```python
from build123d import *

# Parameters (mm, degrees)
SKETCH1_W           = 43.5
SKETCH1_H           = 42.15
SKETCH1_R           = 4
SKETCH1_R_2         = 1
BOSS_EXTRUDE1_DEPTH = 1
BOSS_EXTRUDE2_DEPTH = 3.8
BOSS_EXTRUDE5_DEPTH = 12.8
FILLET1_R           = 1
SKETCH3_R           = 1
CUT_EXTRUDE1_DEPTH  = 63.12336517


with BuildPart() as part:
    # Sketch1 → Boss-Extrude1 (new body)
    with BuildSketch(Plane(origin=(0, 0, 0), x_dir=(1, 0, 0), z_dir=(0, 1, 0))):
        with Locations((21.75, 21.075)):
            Rectangle(SKETCH1_W, SKETCH1_H)
        with Locations(Location((21.75, 21.075, 0), (0, 0, 270))):
            Circle(SKETCH1_R, mode=Mode.SUBTRACT)
        with Locations(Location((21.75, 30.775, 0), (0, 0, 270))):
            Circle(SKETCH1_R, mode=Mode.SUBTRACT)
        with Locations(Location((21.75, 11.375, 0), (0, 0, 90))):
            Circle(SKETCH1_R, mode=Mode.SUBTRACT)
        with Locations(Location((8.55, 21.075, 0), (0, 0, 270))):
            Circle(SKETCH1_R_2, mode=Mode.SUBTRACT)
        with Locations(Location((8.55, 30.725, 0), (0, 0, 270))):
            Circle(SKETCH1_R_2, mode=Mode.SUBTRACT)
        with Locations(Location((8.55, 11.425, 0), (0, 0, 90))):
            Circle(SKETCH1_R_2, mode=Mode.SUBTRACT)
        with Locations(Location((34.95, 11.425, 0), (0, 0, 270))):
            Circle(SKETCH1_R_2, mode=Mode.SUBTRACT)
        with Locations(Location((34.95, 21.075, 0), (0, 0, 90))):
            Circle(SKETCH1_R_2, mode=Mode.SUBTRACT)
        with Locations(Location((34.95, 30.725, 0), (0, 0, 90))):
            Circle(SKETCH1_R_2, mode=Mode.SUBTRACT)
        with Locations(Location((17.012384566, 35.512615434, 0), (0, 0, 270))):
            Circle(SKETCH1_R_2, mode=Mode.SUBTRACT)
        with Locations(Location((17.012384566, 25.812615434, 0), (0, 0, 270))):
            Circle(SKETCH1_R_2, mode=Mode.SUBTRACT)
        with Locations(Location((17.012384566, 16.112615434, 0), (0, 0, 270))):
            Circle(SKETCH1_R_2, mode=Mode.SUBTRACT)
        with Locations(Location((17.012384566, 6.637384566, 0), (0, 0, 270))):
            Circle(SKETCH1_R_2, mode=Mode.SUBTRACT)
        with Locations(Location((26.487615434, 6.637384566, 0), (0, 0, 90))):
            Circle(SKETCH1_R_2, mode=Mode.SUBTRACT)
        with Locations(Location((26.487615434, 16.112615434, 0), (0, 0, 90))):
            Circle(SKETCH1_R_2, mode=Mode.SUBTRACT)
        with Locations(Location((26.487615434, 25.812615434, 0), (0, 0, 90))):
            Circle(SKETCH1_R_2, mode=Mode.SUBTRACT)
        with Locations(Location((26.487615434, 35.512615434, 0), (0, 0, 90))):
            Circle(SKETCH1_R_2, mode=Mode.SUBTRACT)
    extrude(amount=BOSS_EXTRUDE1_DEPTH)

    # Sketch2 → Boss-Extrude2 (add)
    with BuildSketch(Plane(origin=(0, 1, 0), x_dir=(1, 0, 0), z_dir=(0, 1, 0))):
        with BuildLine():
            Line((1, 0.95), (1, 0))
            Line((1, 0), (42.5, 0))
            Line((42.5, 0), (42.5, 0.95))
            ThreePointArc((42.5, 0.95), (42.485355339, 0.985355339), (42.45, 1))
            Line((42.45, 1), (1.05, 1))
            ThreePointArc((1.05, 1), (1.014644661, 0.985355339), (1, 0.95))
        make_face()
        with BuildLine():
            Line((1.05, 41.15), (42.45, 41.15))
            ThreePointArc((42.45, 41.15), (42.485355339, 41.164644661), (42.5, 41.2))
            Line((42.5, 41.2), (42.5, 42.15))
            Line((42.5, 42.15), (1, 42.15))
            Line((1, 42.15), (1, 41.2))
            ThreePointArc((1, 41.2), (1.014644661, 41.164644661), (1.05, 41.15))
        make_face()
    extrude(amount=BOSS_EXTRUDE2_DEPTH)

    # Sketch2<6> → Boss-Extrude5 (add)
    with BuildSketch(Plane(origin=(0, 1, 0), x_dir=(1, 0, 0), z_dir=(0, 1, 0))):
        with BuildLine():
            Line((0.95, 41.15), (0, 41.15))
            Line((0, 41.15), (0, 1))
            Line((0, 1), (0.95, 1))
            ThreePointArc((0.95, 1), (0.985355339, 1.014644661), (1, 1.05))
            Line((1, 1.05), (1, 41.1))
            ThreePointArc((1, 41.1), (0.985355339, 41.135355339), (0.95, 41.15))
        make_face()
        with BuildLine():
            Line((43.5, 1), (43.5, 41.15))
            Line((43.5, 41.15), (42.55, 41.15))
            ThreePointArc((42.55, 41.15), (42.514644661, 41.135355339), (42.5, 41.1))
            Line((42.5, 41.1), (42.5, 1.05))
            ThreePointArc((42.5, 1.05), (42.514644661, 1.014644661), (42.55, 1))
            Line((42.55, 1), (43.5, 1))
        make_face()
    extrude(amount=BOSS_EXTRUDE5_DEPTH)

    # Fillet1
    # the kernel refuses this fillet: 1 mm, written as the material it takes off along each edge
    with BuildSketch(Plane(origin=(42.5, 1, -41.15), x_dir=(1, 0, 0), z_dir=(0, 0, -1))) as fillet1_piece_1_section:
        Polygon((0, 0), (FILLET1_R * 1.02, 0), (FILLET1_R * 1.02, FILLET1_R * 1.02), (0, FILLET1_R * 1.02), align=None)
    fillet1_piece_1 = extrude(amount=FILLET1_R * 1.02, mode=Mode.PRIVATE)
    fillet1_piece_1 = fillet1_piece_1 - Plane(origin=(42.5, 1, -41.15), x_dir=(-0.7071067811865475, 0.7071067811865475, 0), z_dir=(0, 0, -1)) * Sphere(FILLET1_R, mode=Mode.PRIVATE)
    add(fillet1_piece_1, mode=Mode.SUBTRACT)
    with BuildSketch(Plane(origin=(42.5, 1, -1), x_dir=(1, 0, 0), z_dir=(0, 0, 1))) as fillet1_piece_2_section:
        Polygon((0, 0), (FILLET1_R * 1.02, 0), (FILLET1_R * 1.02, -FILLET1_R * 1.02), (0, -FILLET1_R * 1.02), align=None)
    fillet1_piece_2 = extrude(amount=FILLET1_R * 1.02, mode=Mode.PRIVATE)
    fillet1_piece_2 = fillet1_piece_2 - Plane(origin=(42.5, 1, -1), x_dir=(-0.7071067811865475, 0.7071067811865475, 0), z_dir=(0, 0, 1)) * Sphere(FILLET1_R, mode=Mode.PRIVATE)
    add(fillet1_piece_2, mode=Mode.SUBTRACT)
    with BuildSketch(Plane(origin=(1, 1, -1), x_dir=(-1, 0, 0), z_dir=(0, 0, 1))) as fillet1_piece_3_section:
        Polygon((0, 0), (FILLET1_R * 1.02, 0), (FILLET1_R * 1.02, FILLET1_R * 1.02), (0, FILLET1_R * 1.02), align=None)
    fillet1_piece_3 = extrude(amount=FILLET1_R * 1.02, mode=Mode.PRIVATE)
    fillet1_piece_3 = fillet1_piece_3 - Plane(origin=(1, 1, -1), x_dir=(0.7071067811865475, 0.7071067811865475, 0), z_dir=(0, 0, 1)) * Sphere(FILLET1_R, mode=Mode.PRIVATE)
    add(fillet1_piece_3, mode=Mode.SUBTRACT)
    with BuildSketch(Plane(origin=(42.5, 0, -42.15), x_dir=(0, 0, 1), z_dir=(-1, 0, 0))) as fillet1_piece_4:
        with BuildLine():
            CenterArc((FILLET1_R, FILLET1_R), FILLET1_R, 180, 90)
            Line((0, FILLET1_R), (0, 0))
            Line((0, 0), (FILLET1_R, 0))
        make_face()
    extrude(amount=45, mode=Mode.SUBTRACT)
    with BuildSketch(Plane(origin=(43.5, 0, -1), x_dir=(0, 1, 0), z_dir=(0, 0, -1))) as fillet1_piece_5:
        with BuildLine():
            CenterArc((FILLET1_R, -FILLET1_R), FILLET1_R, 90, 90)
            Line((0, -FILLET1_R), (0, 0))
            Line((0, 0), (FILLET1_R, 0))
        make_face()
    extrude(amount=40.15, mode=Mode.SUBTRACT)
    with BuildSketch(Plane(origin=(1, 0, 0), x_dir=(0, 1, 0), z_dir=(1, 0, 0))) as fillet1_piece_6:
        with BuildLine():
            CenterArc((FILLET1_R, -FILLET1_R), FILLET1_R, 90, 90)
            Line((0, -FILLET1_R), (0, 0))
            Line((0, 0), (FILLET1_R, 0))
        make_face()
    extrude(amount=41.5, mode=Mode.SUBTRACT)
    with BuildSketch(Plane(origin=(0, 0, -44.65), x_dir=(0, 1, 0), z_dir=(0, 0, 1))) as fillet1_piece_7:
        with BuildLine():
            CenterArc((FILLET1_R, -FILLET1_R), FILLET1_R, 90, 90)
            Line((0, -FILLET1_R), (0, 0))
            Line((0, 0), (FILLET1_R, 0))
        make_face()
    extrude(amount=43.65, mode=Mode.SUBTRACT)

    # Sketch3 → Cut-Extrude1 (cut, through all)
    with BuildSketch(Plane.ZY):
        with BuildLine():
            ThreePointArc((-3, 13.8), (-1.585786438, 13.214213562), (-1, 11.8))
            Line((-1, 11.8), (-1, 13.8))
            Line((-1, 13.8), (-3, 13.8))
        make_face()
        Polygon((-4, 13.8), (-20, 13.8), (-16, 9.8), (-8, 9.8), align=None)
        with Locations((-19.35, 8.5)):
            Circle(SKETCH3_R)
        with Locations((-23.85, 9.3)):
            Circle(SKETCH3_R)
        with Locations((-31.25, 9.8)):
            Circle(SKETCH3_R)
        with Locations((-38.75, 9.3)):
            Circle(SKETCH3_R)
        with BuildLine():
            Line((-39.15, 13.8), (-41.15, 13.8))
            Line((-41.15, 13.8), (-41.15, 11.8))
            ThreePointArc((-41.15, 11.8), (-40.564213562, 13.214213562), (-39.15, 13.8))
        make_face()
        with Locations((-3.5, 9.3)):
            Circle(SKETCH3_R)
    extrude(amount=-CUT_EXTRUDE1_DEPTH, mode=Mode.SUBTRACT)


solid = part.part
```
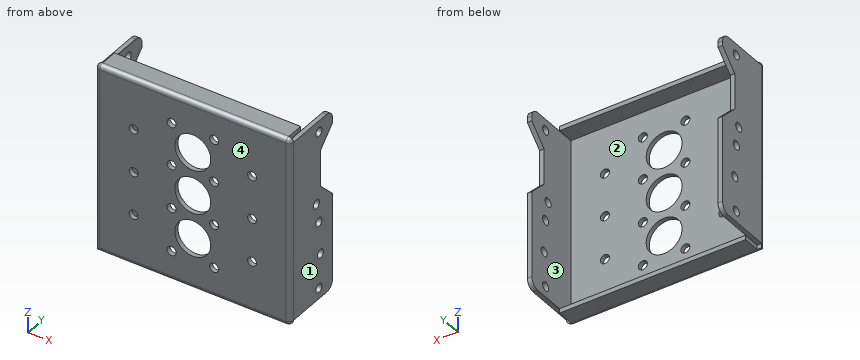
Verification items for the finished model (mm, model axes). Face numbers are marked on the shaded views. Give positions to 0.01 mm unless a question says otherwise; leave off trailing zeros. Write each loop counter-clockwise with the first axis right and the second up, starting at its lowest first coordinate (ties: lowest second). Pieces come first, ordered by that corner, then holes. Notation, with made-up numbers: M -9.5,34.5 L 36.5,34.5 A34 cw 36.5,67.5 Z; hole C 79,-23.5 d10. An arc over 180 degrees is marked long. One line per question, with ' | ' between items.
1) Section check A-A on x = 8.55. Enter the section's corners in (y, z) (3 decimals).
Result:
outline: M 0,-41.15 A1 ccw 1,-42.15 L 4.8,-42.15 L 4.8,-41.15 L 1,-41.15 L 1,-31.725 L 0,-31.725 Z; M 0,-29.725 L 1,-29.725 L 1,-22.075 L 0,-22.075 Z; M 0,-20.075 L 1,-20.075 L 1,-12.425 L 0,-12.425 Z; M 0,-10.425 L 1,-10.425 L 1,-1 L 4.8,-1 L 4.8,0 L 1,0 A1 ccw 0,-1 Z
2) Mould release check, pull along X, two halves, no side actions. Record for the marked faces 1, 2, 3 and 4: released by +X, released by -X, zero draft, split by the parting line, or undercut.
Result:
face 1: released by +X | face 2: undercut | face 3: undercut | face 4: zero draft
3) Section check C-C on z = -3.5. Enter the section's corners in (x, y).
Result:
outline: M 0,1 A1 ccw 1,0 L 42.5,0 A1 ccw 43.5,1 L 43.5,8.3 L 42.5,8.3 L 42.5,1 L 1,1 L 1,8.3 L 0,8.3 Z; M 0,10.3 L 1,10.3 L 1,13.8 L 0,13.8 Z; M 42.5,10.3 L 43.5,10.3 L 43.5,13.8 L 42.5,13.8 Z
4) Section check B-B on y = 2.5. Enter the section's corners in (x, z).
Result:
outline: M 0,-41.15 L 0.95,-41.15 A0.05 ccw 1,-41.1 L 1,-1.05 A0.05 ccw 0.95,-1 L 0,-1 Z; M 1,-42.15 L 42.5,-42.15 L 42.5,-41.2 A0.05 ccw 42.45,-41.15 L 1.05,-41.15 A0.05 ccw 1,-41.2 Z; M 1,-0.95 A0.05 ccw 1.05,-1 L 42.45,-1 A0.05 ccw 42.5,-0.95 L 42.5,0 L 1,0 Z; M 42.5,-41.1 A0.05 ccw 42.55,-41.15 L 43.5,-41.15 L 43.5,-1 L 42.55,-1 A0.05 ccw 42.5,-1.05 Z
5) Thickness scan on line 1 along X through (y, z) = (5.5, -36.5); line 2 along Z through (x, y) = (24.5, 4.25); line 3 along Y through (x, z) = (5, -2). Record the ranges inside material, lowest first. Write a range as [from, to].
Result:
line 1: x = [0, 1], [42.5, 43.5] | line 2: z = [-42.15, -41.15], [-1, 0] | line 3: y = [0, 1]
6) Gauge pin test, flat ends, axial feed: pin 1 Ø0.5 at (y, z) = (2, -41.5) entering from -X; pin 2 Ø10 at (x, z) = (37, -31.5) entering from +Y. Record the tip position at first contact, or that the pin passes through.
Result:
pin 1: stops at x = 1 | pin 2: stops at y = 1
7) Section check D-D on y = 5.75. Enter the section's corners in (x, z), plus the area to 3 significant figures.
Result:
outline: M 0,-41.15 L 0.95,-41.15 A0.05 ccw 1,-41.1 L 1,-1.05 A0.05 ccw 0.95,-1 L 0,-1 Z; M 42.5,-41.1 A0.05 ccw 42.55,-41.15 L 43.5,-41.15 L 43.5,-1 L 42.55,-1 A0.05 ccw 42.5,-1.05 Z | area: 80.3 mm2
